from build123d import *

# Parameters (mm, degrees)
CUT_EXTRUDE1_START = -16
CUT_EXTRUDE1_DEPTH = 16


with BuildPart() as part:
    # Sketch1 → Revolve1 (revolve)
    with BuildSketch(Plane(origin=(0, 0, 0), x_dir=(1, 0, 0), z_dir=(0, 1, 0)), mode=Mode.PRIVATE) as revolve1_sk:
        Polygon((15, 0), (30, 0), (30, 5), (20, 5), (20, 35), (30, 35), (30, 40), (14, 40), (14, 16), (15, 16), align=None)
    revolve(revolve1_sk.sketch.rotate(Axis((0, 0, -89.857142857), (0, 0, 1)), 180), axis=Axis((0, 0, -89.857142857), (0, 0, 1)))

    # Sketch2 → Cut-Extrude1 (cut)
    with BuildSketch(Plane(origin=(0, 0, -40), x_dir=(-1, 0, 0), z_dir=(0, 0, -1)).offset(CUT_EXTRUDE1_START)):
        with BuildLine():
            Line((4, 17.3), (-4, 17.3))
            Line((-4, 17.3), (-4, 13.416407865))
            ThreePointArc((-4, 13.416407865), (0, 14), (4, 13.416407865))
            Line((4, 13.416407865), (4, 17.3))
        make_face()
    extrude(amount=CUT_EXTRUDE1_DEPTH, mode=Mode.SUBTRACT)


solid = part.part
Geometry: final body of the model. Coordinates: model frame, mm. A direction names the side the tool comes from. Round coordinates to 2 decimals unless told otherwise and drop trailing zeros. Order: outer loops, then holes, each group sorted by start corner. A loop starts at its lowest first (then second) coordinate and runs counter-clockwise, first axis right, second up.
Q1. Section C-C, the plane z = -32. Output: boundary loops of the cut face in (x, y), and give its area (3 significant figures).
Result sheet:
outline: circle Ø40 at (0, 0); hole (-4, 13.42) arc R14 ccw (long way) to (4, 13.42) - (4, 17.3) - (-4, 17.3) - close
area: 613 mm2
Q2. Section D-D, the plane x = -6. Output: boundary loops of the cut face in (y, z).
Result sheet:
outline: (-29.39, -40) - (-12.65, -40) - (-12.65, -16) - (-13.75, -16) - (-13.75, 0) - (-29.39, 0) - (-29.39, -5) - (-19.08, -5) - (-19.08, -35) - (-29.39, -35) - close; (12.65, -40) - (29.39, -40) - (29.39, -35) - (19.08, -35) - (19.08, -5) - (29.39, -5) - (29.39, 0) - (13.75, 0) - (13.75, -16) - (12.65, -16) - close
Q3. Section B-B, the plane y = 7. Output: boundary loops of the cut face in (x, z) (1 decimal).
Result sheet:
outline: (-29.2, -40) - (-12.1, -40) - (-12.1, -16) - (-13.3, -16) - (-13.3, 0) - (-29.2, 0) - (-29.2, -5) - (-18.7, -5) - (-18.7, -35) - (-29.2, -35) - close; (12.1, -40) - (29.2, -40) - (29.2, -35) - (18.7, -35) - (18.7, -5) - (29.2, -5) - (29.2, 0) - (13.3, 0) - (13.3, -16) - (12.1, -16) - close
Q4. Material intervals for probe 1 along Y at (x, z) = (0, -6); probe 2 along Z at (x, y) = (-17, -21); probe 3 along Y at (x, z) = (0, -3.25), sorted ascending.
Result sheet:
probe 1: y = -20 to -15, 15 to 20
probe 2: z = -40 to -35, -5 to 0
probe 3: y = -30 to -15, 15 to 30
Q5. Mould query, pull axis Z, two halves, no side actions, for faces 1 (the face through (0, 15, -24)), 2 (the face through (-6, 20, -5)), 3 (the face through (-16.128, -25.296, -37.535)). Classes: released by +Z, released by -Z, zero draft, split by the parting line, or undercut.
Result sheet:
face 1: released by -Z
face 2: undercut
face 3: zero draft
Q6. Pin query (flat end, axial travel): pin 1 (3 mm diameter, centred on x = 0.5, y = 15, fed in from -Z); pin 2 (9 mm diameter, centred on x = 1.5, z = -33, fed in from -Y); pin 3 (2 mm diameter, centred on y = -21.5, z = -29.5, fed in from +X); pin 4 (6 mm diameter, centred on x = -21, z = -36, fed in from -Y). Return the tip coordinate at first contact, or that it passes through.
Result sheet:
pin 1: stops at z = -24
pin 2: stops at y = -30
pin 3: passes through
pin 4: stops at y = -24
Q7. Section A-A, the plane x = 0. Output: boundary loops of the cut face in (y, z), and give its area (3 significant figures).
Result sheet:
outline: (-30, -40) - (-14, -40) - (-14, -16) - (-15, -16) - (-15, 0) - (-30, 0) - (-30, -5) - (-20, -5) - (-20, -35) - (-30, -35) - close; (14, -24) - (17.3, -24) - (17.3, -40) - (30, -40) - (30, -35) - (20, -35) - (20, -5) - (30, -5) - (30, 0) - (15, 0) - (15, -16) - (14, -16) - close
area: 595 mm2
Q8. Access query for faces 4 (the face through (0, 17.3, -32)), 5 (the face through (6, -14, 0)), 6 (the face through (19.98, -0.88, -20.21)), 7 (the face through (-8.06, -12.65, -7.89)), 8 (the face through (-16.128, -25.296, -2.535)). Directions: +Z, -Z, +X, -X, +Y, -Y. A direction counts if a zero-diameter tool reaches every point of the face in a straight line with its end or side. Return the directions, or none.
Result sheet:
face 4: -Z
face 5: +Z, +X, -X, +Y, -Y
face 6: none
face 7: +Z
face 8: +Z, -Z
